Verification items for the finished model (mm, model axes). A direction names the side the tool comes from. Coordinates: 2 decimals unless noted, no trailing zeros. Order: outer loops, then holes, each group sorted by start corner. A loop starts at its lowest first (then second) coordinate and runs counter-clockwise, first axis right, second up. Notation, with made-up numbers: (39.5, 50.25) -> (91.5, 50.25) arc R36 cw to (91.5, 88.25) -> close; hole circle Ø1 at (35.5, 87). An arc over 180 degrees is marked (long way). Write item = value, one per line. Start each with the question number.
1. Cross-section at C-C on x = 4.5. Record the cut outline in (y, z), plus the area to 3 significant figures.
2. Thickness scan on line 1 along Z through (x, y) = (8.5, 53); line 2 along Y through (x, z) = (20, 77.3); line 3 along Y through (x, z) = (12.5, 36). Record the ranges inside material, lowest first. Write a range as from..to.
3. Cross-section at D-D on z = 31. Record the cut outline in (x, y), plus the area to 3 significant figures.
4. Set-up check for faces 4 (the flat face through (20, 80, 38)), 5 (the flat face through (20, 39, 1)): record each of +Z, -Z, +X, -X, +Y, -Y from which the full face is reachable in a straight line by a thin tool's end or side.
5. Release check for a two-part mould opening along Y. For faces 1 (the flat face through (20, 79, 38)), 2 (the cylindrical face through (18.41, 9.9, 77.51)), 3 (the flat face through (20, 39, 0)) record: +Y half, -Y half, draft (parallel to the pull), parting line (faces both ways), or undercut.
6. Cross-section at A-A on y = 63.5. Record the cut outline in (x, z).
7. Go/stop test with flat-tipped pins: P1, Ø6.5, axis at x = 20, y = 11.11, coming from the -Z side; P2, Ø5, axis at x = 27.5, z = 9.5, coming from the -Y side. Record where each tip stops, or that it passes through.
8. Cross-section at B-B on x = 20. Record the cut outline in (y, z), plus the area to 3 significant figures.
Autodesk Inventor part; units mm, degrees
ref_plane "YZ Plane" through (0, 0, 0) normal (1, 0, 0) x (0, 1, 0)
ref_plane "XZ Plane" through (0, 0, 0) normal (0, 1, 0) x (-1, 0, 0)
ref_plane "XY Plane" through (0, 0, 0) normal (0, 0, 1) x (1, 0, 0)
sketch "Sketch2" plane through (0, 0, 0) normal (1, 0, 0) x (0, 1, 0)
  line L0 (0, 0) -> (80, 0)
  line L1 (80, 0) -> (80, 78)
  line L2 (80, 78) -> (0, 78)
  line L3 (0, 78) -> (0, 0)
  dimension "d3" = 80
  dimension "d4" = 78
extrude "Extrusion2" add sketch "Sketch2" along normal blind 40
shell "Shell1" thickness 1 removed faces 3 at (13.3333, 0, 52) at (0, 26.6667, 52) at (40, 26.6667, 52)
sketch "Sketch3" plane through (0, 0, 78) normal (0, 0, 1) x (1, 0, 0)
  line L0 (0, 0) -> (40, 0)
  line L1 (0, 80) -> (40, 80)
  circle A0 centre (20, 11.1124) radius 2
  dimension "d8" = 4
extrude "Extrusion3" cut sketch "Sketch3" against normal blind 1
properties part number "MAN_BASIS_SECONDARY_STRUCTURE"
Worked out:
q1.outline = (0, 0) -> (80, 0) -> (80, 78) -> (0, 78) -> (0, 77) -> (79, 77) -> (79, 1) -> (0, 1) -> close
q1.area = 236 mm²
q2.line_1 = 0..1, 77..78
q2.line_2 = 0..9.11, 13.11..80
q2.line_3 = 79..80
q3.outline = (0, 79) -> (40, 79) -> (40, 80) -> (0, 80) -> close
q3.area = 40.0 mm²
q4.face_4 = +Z, -Z, +X, -X, +Y
q4.face_5 = +X, -X, -Y
q5.face_1 = -Y half
q5.face_2 = undercut
q5.face_3 = draft
q6.outline = (0, 0) -> (40, 0) -> (40, 1) -> (0, 1) -> close; (0, 77) -> (40, 77) -> (40, 78) -> (0, 78) -> close
q7.P1 = 0
q7.P2 = 79
q8.outline = (0, 0) -> (80, 0) -> (80, 78) -> (13.11, 78) -> (13.11, 77) -> (79, 77) -> (79, 1) -> (0, 1) -> close; (0, 77) -> (9.11, 77) -> (9.11, 78) -> (0, 78) -> close
q8.area = 232 mm²
